Can you work these out from the model? Positions are in its coordinate system, mm. Face numbers are marked on the shaded views. A direction names the side the tool comes from. Round coordinates to 2 decimals unless told otherwise and drop trailing zeros. Order: outer loops, then holes, each group sorted by start corner. A loop starts at its lowest first (then second) coordinate and runs counter-clockwise, first axis right, second up. Notation, with made-up numbers: (19.25, 30.5) -> (33.25, 30.5) arc R23 cw to (33.25, 69.5) -> close; hole circle Ø2 at (-30.75, -34.75). An arc over 180 degrees is marked (long way). One line per item, written item: value.
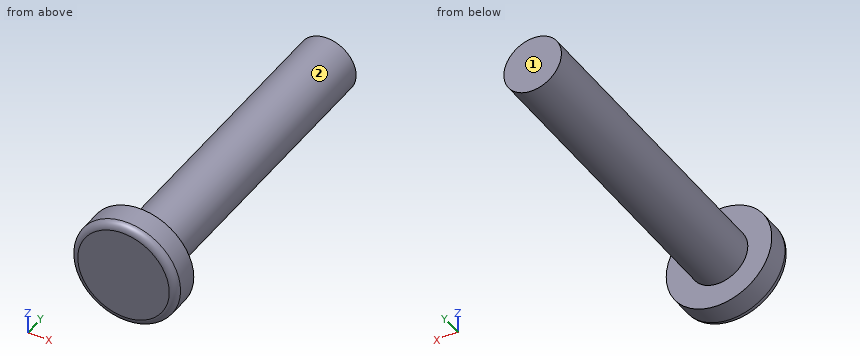
```python
from build123d import *

# Parameters (mm, degrees)
SKETCH_1_W      = 2.75
SKETCH_1_H      = 1.5
SKETCH_2_R      = 1.5
EXTRUDE_1_DEPTH = 16
FILLET_1_R      = 0.367346939


with BuildPart() as part:
    # 草图1 → 旋转1 (revolve)
    with BuildSketch(Plane.XY.offset(15)):
        with Locations((1.375, 0.75)):
            Rectangle(SKETCH_1_W, SKETCH_1_H)
    revolve(axis=Axis((0, 1.5, 15), (0, -1, 0)))

    # 草图2 → 凸台-拉伸1 (add)
    with BuildSketch(Plane(origin=(0, 1.5, 0), x_dir=(-1, 0, 0), z_dir=(0, 1, 0))):
        with Locations((0, 15)):
            Circle(SKETCH_2_R)
    extrude(amount=EXTRUDE_1_DEPTH)

    # 圆角1
    fillet_1_edges = [part.edges().sort_by_distance(p)[0] for p in [
        (-2.75, 0, 15),
    ]]
    fillet(fillet_1_edges, radius=FILLET_1_R)


solid = part.part
```
Q1. I want a section at B-B on x = 0. List the corners of the cut face in (y, z) for me, plus the area to 3 significant figures.
Answers below:
outline: (0, 12.62) arc R0.37 ccw to (0.37, 12.25) -> (1.5, 12.25) -> (1.5, 13.5) -> (17.5, 13.5) -> (17.5, 16.5) -> (1.5, 16.5) -> (1.5, 17.75) -> (0.37, 17.75) arc R0.37 ccw to (0, 17.38) -> close
area: 56.2 mm^2
Q2. On a 3-axis mill with a long thin cutter (end or side, diameter ignored), from which of +Z, -Z, +X, -X, +Y, -Y can I reach the whole of each face in a straight line? I mean the marked faces 1 and 2. Say none if no direction works.
Answers below:
face 1: +Z, -Z, +X, -X, +Y
face 2: +Y
Q3. I want a section at A-A on z = 15. List the corners of the cut face in (x, y) for me.
Answers below:
outline: (-2.75, 0.37) arc R0.37 ccw to (-2.38, 0) -> (2.38, 0) arc R0.37 ccw to (2.75, 0.37) -> (2.75, 1.5) -> (1.5, 1.5) -> (1.5, 17.5) -> (-1.5, 17.5) -> (-1.5, 1.5) -> (-2.75, 1.5) -> close
Q4. I want a section at C-C on y = 3. List the corners of the cut face in (x, z) for me, plus the area to 3 significant figures.
Answers below:
outline: circle Ø3 at (0, 15)
area: 7.07 mm^2
Q5. Please list where these lines run through material, in increasing order: line 1 along Y through (x, z) = (-0.25, 16.6); line 2 along Z through (x, y) = (0, 7.25); line 3 along Z through (x, y) = (1.2, 9.75).
Answers below:
line 1: 0 to 1.5
line 2: 13.5 to 16.5
line 3: 14.1 to 15.9
Q6. Will these pins go through, and if not, where does the flat tip stop? pin 1 Ø1.5 at (y, z) = (8, 16.5) entering from +X; pin 2 Ø3 at (y, z) = (9.5, 15) entering from +X; pin 3 Ø1 at (y, z) = (5.5, 16) entering from -X; pin 4 Ø3 at (x, z) = (0.5, 16) entering from -Y.
Answers below:
pin 1: x = 1.3
pin 2: x = 1.5
pin 3: x = -1.41
pin 4: y = 0
